For this review, take the finished solid that the model builds, in its own axes (mm). Give positions to 0.01 mm unless a question says otherwise; leave off trailing zeros. Loops run counter-clockwise (first coordinate to the right, second up) from the corner with the lowest first, then second, coordinate; pieces in that order, holes last.
```python
from build123d import *

# Parameters (mm, degrees)
SKETCH1_R          = 55
EXTRUDE_3_8_DEPTH  = 10
SKETCH5_R          = 6.35
CUT_EXTRUDE2_DEPTH = 10
SKETCH6_R          = 2.2
M4_THROUGH2_DEPTH  = 10
SKETCH7_R          = 2.75
CUT_EXTRUDE4_DEPTH = 10


with BuildPart() as part:
    # Sketch1 → 3/8 (new body)
    with BuildSketch(Plane.XY):
        Circle(SKETCH1_R)
    extrude(amount=EXTRUDE_3_8_DEPTH)

    # Sketch5 → Cut-Extrude2 (cut)
    with BuildSketch(Plane.XY.offset(10)):
        Circle(SKETCH5_R)
    extrude(amount=-CUT_EXTRUDE2_DEPTH, mode=Mode.SUBTRACT)

    # Sketch6 → M4_through2 (cut)
    with BuildSketch(Plane.XY.offset(10)):
        with Locations((0, 15)):
            Circle(SKETCH6_R)
        with Locations((0, -15)):
            Circle(SKETCH6_R)
    extrude(amount=-M4_THROUGH2_DEPTH, mode=Mode.SUBTRACT)

    # Sketch7 → Cut-Extrude4 (cut)
    with BuildSketch(Plane.XY.offset(10)):
        with Locations((-40, 0)):
            Circle(SKETCH7_R)
    extrude(amount=-CUT_EXTRUDE4_DEPTH, mode=Mode.SUBTRACT)


solid = part.part
```
Q1. For probe 1 along Y at (x, z) = (0, 4.25); probe 2 along X at (y, z) = (-1, 7.75); probe 3 along Y at (x, z) = (-40, 6.5), list the stretches that pass through material, from the lowest coordinate up.
Answers:
probe 1: y = -55 to -17.2, -12.8 to -6.35, 6.35 to 12.8, 17.2 to 55
probe 2: x = -54.99 to -42.56, -37.44 to -6.27, 6.27 to 54.99
probe 3: y = -37.75 to -2.75, 2.75 to 37.75
Q2. Consider section B-B on z = 6.25. Give the boundary of the cut face in (x, y).
Answers:
outline: circle Ø110 at (0, 0); hole circle Ø5.5 at (-40, 0); hole circle Ø12.7 at (0, 0); hole circle Ø4.4 at (0, -15); hole circle Ø4.4 at (0, 15)
Q3. For pin 1 Ø4 at (x, y) = (-16.5, 2) entering from -Z; pin 2 Ø1 at (x, z) = (31.5, 5) entering from -Y; pin 3 Ø4 at (y, z) = (42, 2.5) entering from -X; pin 4 Ø2.5 at (x, y) = (0, 15) entering from -Z, all flat-tipped, find the tip position at first contact; note any pin that passes through.
Answers:
pin 1: stops at z = 0
pin 2: stops at y = -45.43
pin 3: stops at x = -37.75
pin 4: passes through
Q4. Mouldability with a two-part tool opening along Y and no side actions: class faces 1 (the cylindrical face through (-11.923, -53.692, 4.93)), 2 (the flat face through (11, 1, 0)), 3 (the cylindrical face through (-2.198, 15.097, 5.07)) as +Y half, -Y half, draft (parallel to the pull), parting line (faces both ways), or undercut.
Answers:
face 1: parting line
face 2: draft
face 3: undercut
Q5. Consider section A-A on y = 0. Give the boundary of the cut face in (x, z), plus the area to 3 significant figures.
Answers:
outline: (-55, 0) - (-42.75, 0) - (-42.75, 10) - (-55, 10) - close; (-37.25, 0) - (-6.35, 0) - (-6.35, 10) - (-37.25, 10) - close; (6.35, 0) - (55, 0) - (55, 10) - (6.35, 10) - close
area: 918 mm2
Q6. Consider section C-C on x = -40. Give the boundary of the cut face in (y, z).
Answers:
outline: (-37.75, 0) - (-2.75, 0) - (-2.75, 10) - (-37.75, 10) - close; (2.75, 0) - (37.75, 0) - (37.75, 10) - (2.75, 10) - close
Q7. Consider section D-D on y = -15. Give the boundary of the cut face in (x, z), plus the area to 3 significant figures.
Answers:
outline: (-52.92, 0) - (-2.2, 0) - (-2.2, 10) - (-52.92, 10) - close; (2.2, 0) - (52.92, 0) - (52.92, 10) - (2.2, 10) - close
area: 1,010 mm2
